Here's the drawing with two shaded views (mm, measured from the low corner). I have some questions. Coordinates: 2 decimals unless noted, no trailing zeros. Write each loop counter-clockwise with the first axis right and the second up, starting at its lowest first coordinate (ties: lowest second). Pieces come first, ordered by that corner, then holes. Notation, with made-up numbers: (9.5, 2.25) -> (30.5, 2.25) arc R11 cw to (30.5, 11.25) -> close; hole circle Ø9 at (57.25, 8). An arc over 180 degrees is marked (long way). Answer in a Markdown table with one row per item. Add a question column.
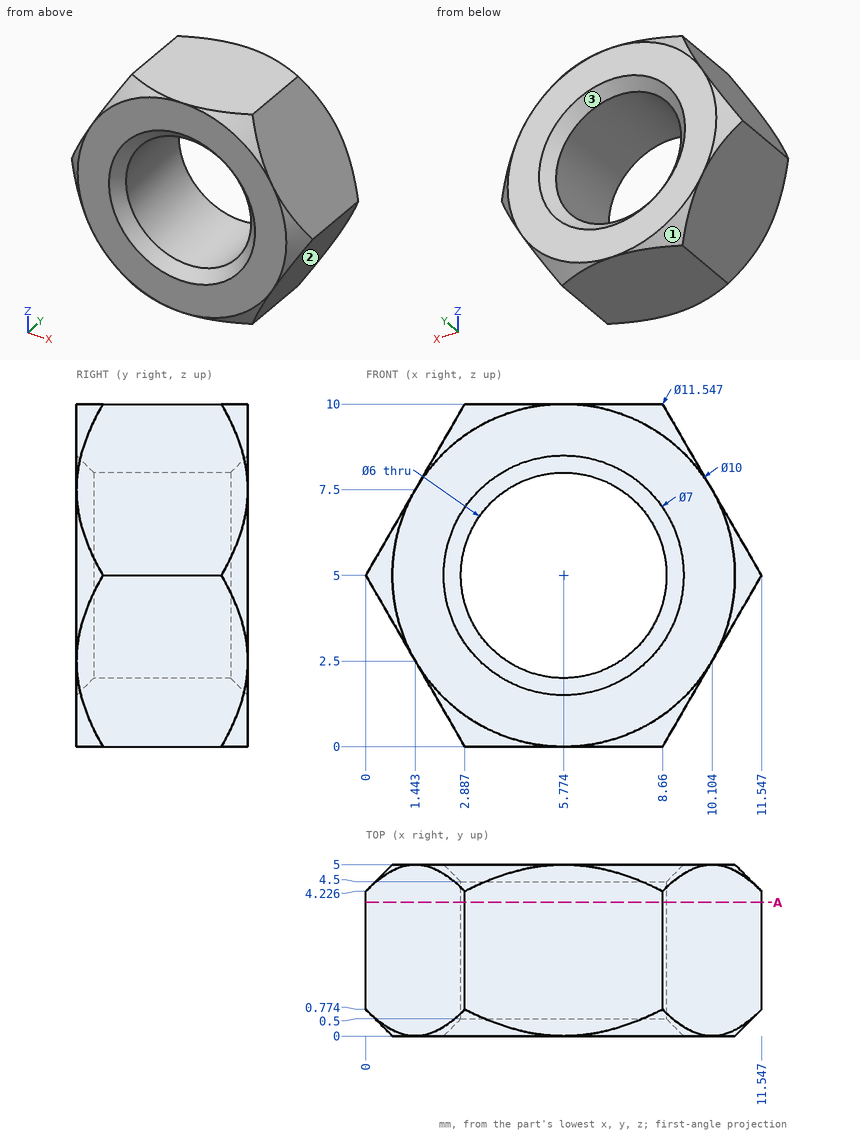
Q1. Imagine slicing it at A-A on y = 3.9. Please give me the cut outline in (x, z).
Q2. If we mould it in two halves opening along X, with no side actions, what happens to the marked faces 1, 2 and 3? For each: pulls with the +X half, pulls with the -X half, needs draft (parallel to the pull), parting line crosses it, or undercut.
Q3. I need wall thicknesses on line 1 (X direction, y = 2.15, z = 6.5) (1 decimal); line 2 (X direction, y = 1.8, z = 6.25) (1 decimal); line 3 (Z direction, x = 8, y = 1.85). Which ranges of each line are inside material? Lowest first, please. Write a range as [from, to].
Q4. I'm going to push flat-ended pins straight in: P1, Ø1.5, axis at x = 1.5, y = 3.5, coming from the -Z side (1 decimal); P2, Ø1.5, axis at x = 1.5, y = 1, coming from the +Z side (1 decimal); P3, Ø1.5, axis at x = 2, y = 2.5, coming from the -Z side (1 decimal). Where does each tip first touch, or does it pass through?
Result sheet:
| question | item | result |
|---|---|---|
| 1 | outline | (0, 5) -> (2.89, 0) -> (8.66, 0) -> (11.55, 5) -> (8.66, 10) -> (2.89, 10) -> close; hole circle Ø6 at (5.77, 5) |
| 2 | face 1 | pulls with the -X half |
| 2 | face 2 | pulls with the +X half |
| 2 | face 3 | undercut |
| 3 | line 1 | x = [0.9, 3.2], [8.4, 10.7] |
| 3 | line 2 | x = [0.7, 3], [8.5, 10.8] |
| 3 | line 3 | z = [0, 2.99], [7.01, 10] |
| 4 | P1 | stops at z = 1.1 |
| 4 | P2 | stops at z = 8.9 |
| 4 | P3 | stops at z = 0.2 |
